```python
from build123d import *

# Parameters (mm, degrees)
SKETCH_1_W          = 10
SKETCH_1_H          = 10
SKETCH_1_W_2        = 8
SKETCH_1_H_2        = 8
EXTRUDE_1_DEPTH     = 67
CUT_EXTRUDE_1_REACH = 70.476
SKETCH_2_R          = 1.6
CUT_EXTRUDE_2_REACH = 70.476
SKETCH_3_R          = 4
SKETCH_3_R_2        = 3


with BuildPart() as part:
    # ｽｹｯﾁ1 → 押し出し-薄板1 (new body)
    with BuildSketch(Plane(origin=(0, 0, 0), x_dir=(1, 0, 0), z_dir=(0, 1, 0))):
        with Locations((5, 5)):
            Rectangle(SKETCH_1_W, SKETCH_1_H)
        with Locations((5, 5)):
            Rectangle(SKETCH_1_W_2, SKETCH_1_H_2, mode=Mode.SUBTRACT)
    extrude(amount=EXTRUDE_1_DEPTH)

    # ｶｯﾄ - 押し出し1: up to this face of the body (flat: up to its plane)
    cut_extrude_1_end = Plane(part.part.faces().sort_by_distance((5, 33.5, -10))[0])
    # ｽｹｯﾁ2 → ｶｯﾄ - 押し出し1 (cut, up to the picked face)
    with BuildSketch(Plane.XY, mode=Mode.PRIVATE) as cut_extrude_1_sk1:
        with Locations((5, 62)):
            Circle(SKETCH_2_R)
    cut_extrude_1_tool1 = split(extrude(cut_extrude_1_sk1.sketch, amount=-CUT_EXTRUDE_1_REACH, mode=Mode.PRIVATE), bisect_by=cut_extrude_1_end, keep=Keep.BOTH, mode=Mode.PRIVATE)
    add(cut_extrude_1_tool1.solids().sort_by(Axis((5, 62, 0), (0, 0, -1)))[0], mode=Mode.SUBTRACT)

    # ｶｯﾄ - 押し出し2: up to this face of the body (flat: up to its plane)
    cut_extrude_2_end = Plane(part.part.faces().sort_by_distance((0, 33.5, -5))[0])
    # ｽｹｯﾁ3 → ｶｯﾄ - 押し出し2 (cut, up to the picked face)
    with BuildSketch(Plane(origin=(10, 0, 0), x_dir=(0, 0, -1), z_dir=(1, 0, 0)), mode=Mode.PRIVATE) as cut_extrude_2_sk1:
        with Locations((5, 62)):
            Circle(SKETCH_3_R)
    cut_extrude_2_tool1 = split(extrude(cut_extrude_2_sk1.sketch, amount=-CUT_EXTRUDE_2_REACH, mode=Mode.PRIVATE), bisect_by=cut_extrude_2_end, keep=Keep.BOTH, mode=Mode.PRIVATE)
    # ｽｹｯﾁ3 → ｶｯﾄ - 押し出し2 (cut, up to the picked face)
    with BuildSketch(Plane(origin=(10, 0, 0), x_dir=(0, 0, -1), z_dir=(1, 0, 0)), mode=Mode.PRIVATE) as cut_extrude_2_sk2:
        with Locations((5, 5)):
            Circle(SKETCH_3_R_2)
    cut_extrude_2_tool2 = split(extrude(cut_extrude_2_sk2.sketch, amount=-CUT_EXTRUDE_2_REACH, mode=Mode.PRIVATE), bisect_by=cut_extrude_2_end, keep=Keep.BOTH, mode=Mode.PRIVATE)
    add(cut_extrude_2_tool1.solids().sort_by(Axis((10, 62, -5), (-1, 0, 0)))[0], mode=Mode.SUBTRACT)
    add(cut_extrude_2_tool2.solids().sort_by(Axis((10, 5, -5), (-1, 0, 0)))[0], mode=Mode.SUBTRACT)


solid = part.part
```
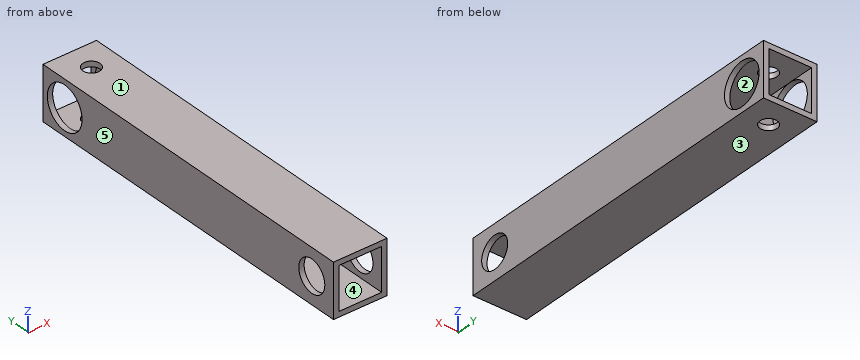
For this review, take the finished solid that the model builds, in its own axes (mm). Face numbers are marked on the shaded views. A direction names the side the tool comes from. Coordinates: 2 decimals unless noted, no trailing zeros. Write each loop counter-clockwise with the first axis right and the second up, starting at its lowest first coordinate (ties: lowest second). Pieces come first, ordered by that corner, then holes. Notation, with made-up numbers: (42.25, 5.5) - (62.25, 5.5) arc R29 cw to (62.25, 37.5) - close; hole circle Ø4 at (67.5, -27.75). An arc over 180 degrees is marked (long way). Put each result on its own line as item: value.
1. Wall thickness on probe 1 along Y at (x, z) = (9.2, -5); probe 2 along X at (y, z) = (62, -9.6); probe 3 along X at (y, z) = (22.5, -3.5): over which ranges is each line inside the solid? List them lowest first.
Values found:
probe 1: 0 to 2, 8 to 58, 66 to 67
probe 2: 0 to 3.4, 6.6 to 10
probe 3: 0 to 1, 9 to 10
2. Mouldability with a two-part tool opening along X and no side actions: class the marked faces 3, 4 and 5 as released by +X, released by -X, zero draft, split by the parting line, or undercut.
Values found:
face 3: zero draft
face 4: undercut
face 5: released by -X
3. Machinability: for the marked faces 1 and 2, which of the approach directions +Z, -Z, +X, -X, +Y, -Y give a long, thin tool a straight path to every point of the face, cutting with its end or side? Answer none if there is none.
Values found:
face 1: +Z, +X, -X, +Y, -Y
face 2: +Y, -Y
4. Add section A-A, the plane x = 5. Give the boundary of the cut face in (y, z), then the cut area to 3 significant figures.
Values found:
outline: (0, -10) - (60.4, -10) - (60.4, -9) - (0, -9) - close; (0, -1) - (60.4, -1) - (60.4, 0) - (0, 0) - close; (63.6, -10) - (67, -10) - (67, -9) - (63.6, -9) - close; (63.6, -1) - (67, -1) - (67, 0) - (63.6, 0) - close
area: 128 mm²
5. Add section C-C, the plane y = 31.5. Give the boundary of the cut face in (x, z), then the cut area to 3 significant figures.
Values found:
outline: (0, -10) - (10, -10) - (10, 0) - (0, 0) - close; hole (1, -9) - (9, -9) - (9, -1) - (1, -1) - close
area: 36.0 mm²
6. Add section B-B, the plane z = -5. Give the boundary of the cut face in (x, y).
Values found:
outline: (0, 0) - (1, 0) - (1, 2) - (0, 2) - close; (0, 8) - (1, 8) - (1, 58) - (0, 58) - close; (0, 66) - (1, 66) - (1, 67) - (0, 67) - close; (9, 0) - (10, 0) - (10, 2) - (9, 2) - close; (9, 8) - (10, 8) - (10, 58) - (9, 58) - close; (9, 66) - (10, 66) - (10, 67) - (9, 67) - close
